Part model, mm, in its own coordinate system. Face numbers are marked on the shaded views. A direction names the side the tool comes from. Give positions to 0.01 mm unless a question says otherwise; leave off trailing zeros. Write each loop counter-clockwise with the first axis right and the second up, starting at its lowest first coordinate (ties: lowest second). Pieces come first, ordered by that corner, then holes. Notation, with made-up numbers: M -29,-19.75 L -17,-19.75 A22 cw -17,0.25 Z; hole C 66,-30 d9. An arc over 180 degrees is marked long. Answer as CSV lines item,"result". Start each with the question number.
Item 1: Band-saw the part on C-C, the plane z = -19.5. List the corners of the cut face in (x, y), then the cut area to 3 significant figures.
Item 2: Band-saw the part on D-D, the plane z = 14. List the corners of the cut face in (x, y), then the cut area to 3 significant figures.
Item 3: 3-axis set-ups, long thin cutter, end or side, ignore diameter. For the marked faces 4, 5 and 6: which of +Z, -Z, +X, -X, +Y, -Y reach the whole face in a straight line?
Item 4: Two-plate mould, pull along X, no slides. Class the marked faces 1, 2 and 3: +X half, -X half, draft (parallel to the pull), parting line (faces both ways), or undercut.
Item 5: Pin check, flat tips, straight feed: pin 1 (4 mm diameter, centred on x = 104.5, y = 0.5, fed in from +Z); pin 2 (1.2 mm diameter, centred on x = 89.5, y = -1.5, fed in from +Z); pin 3 (3 mm diameter, centred on y = -1.5, z = 1, fed in from +X); pin 4 (3 mm diameter, centred on x = 84, y = -0.5, fed in from +Z). Stop position of each tip, or through.
Item 6: Band-saw the part on B-B, the plane y = 2. List the corners of the cut face in (x, z) (3 decimals), then the cut area to 3 significant figures.
Item 7: Wall check: L1, parallel to X at y = 1.5, z = -7; L2, parallel to Z at x = 100, y = -1; L3, parallel to Y at x = 92, z = -19. Give the ranges that are in metal, low to high. Write a range as from..to.
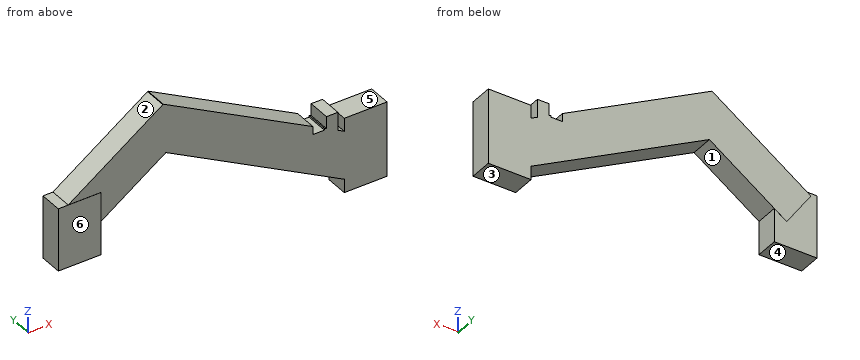
from build123d import *

# Parameters (mm, degrees)
F4_W      = 8
F4_H      = 15
F5_DEPTH  = 41.9
F6_W      = 8
F6_H      = 15
F7_DEPTH  = 84.2
F8_DEPTH  = 4.9
F9_W      = 15
F9_H      = 8
F10_DEPTH = 15.3
F11_DEPTH = 6.8
F12_W     = 15
F12_H     = 8
F13_DEPTH = 26.4
F14_W     = 4
F14_H     = 8
F15_DEPTH = 1.5
F16_W     = 4
F16_H     = 8
F17_DEPTH = 5
F18_DEPTH = 3


with BuildPart() as f5:
    # F4 (on face) → F5 (new body)
    with BuildSketch(Plane(origin=(-0.447452, 0, -0.306762), x_dir=(0, 1, 0), z_dir=(0.824783, 0, 0.56545))):
        Rectangle(F4_W, F4_H)
    extrude(amount=F5_DEPTH)

    # F6 (on face) → F7 (join)
    with BuildSketch(Plane(origin=(15.159437, 0, -8.175749), x_dir=(0, -1, 0), z_dir=(-0.880156, 0, 0.474684))):
        with Locations((0, 32.858156)):
            Rectangle(F6_W, F6_H)
    extrude(amount=-F7_DEPTH)

    # F6 (on face) → F8 (join)
    with BuildSketch(Plane(origin=(15.159437, 0, -8.175749), x_dir=(0, -1, 0), z_dir=(-0.880156, 0, 0.474684))):
        with Locations((0, 32.858156)):
            Rectangle(F6_W, F6_H)
    extrude(amount=F8_DEPTH)

    # F9 (on Top) → F10 (join)
    with BuildSketch(Plane.XY):
        with Locations((0.658734, -0.029655)):
            Rectangle(F9_W, F9_H)
    extrude(amount=-F10_DEPTH)

    # F9 (on Top) → F11 (join)
    with BuildSketch(Plane.XY):
        with Locations((0.658734, -0.029655)):
            Rectangle(F9_W, F9_H)
    extrude(amount=F11_DEPTH)

    # F12 (on Top) → F13 (join)
    with BuildSketch(Plane.XY):
        with Locations((101.044647, 0)):
            Rectangle(F12_W, F12_H)
    extrude(amount=-F13_DEPTH)

    # F14 (on Top) → F15 (cut, symmetric)
    with BuildSketch(Plane.XY):
        with Locations((84.574081, 0)):
            Rectangle(F14_W, F14_H)
    extrude(amount=F15_DEPTH, both=True, mode=Mode.SUBTRACT)

    # F16 (on Top) → F17 (join)
    with BuildSketch(Plane.XY):
        with Locations((89.305073, 0)):
            Rectangle(F16_W, F16_H)
    extrude(amount=-F17_DEPTH)

    # F16 (on Top) → F18 (join)
    with BuildSketch(Plane.XY):
        with Locations((89.305073, 0)):
            Rectangle(F16_W, F16_H)
    extrude(amount=F18_DEPTH)


solid = f5.part
Output:
1,outline,"M 89.58,-4 L 108.54,-4 L 108.54,4 L 89.58,4 Z"
1,area,"152 mm²"
2,outline,"M 7.16,-4 L 59.06,-4 L 59.06,4 L 7.16,4 Z"
2,area,"415 mm²"
3,face 4,"-Z, -X, +Y, -Y"
3,face 5,"+Z, +X, +Y, -Y"
3,face 6,"+Z, -Z, +X, -X, -Y"
4,face 1,"undercut"
4,face 2,"-X half"
4,face 3,"draft"
5,pin 1,"z = 0"
5,pin 2,"z = 3"
5,pin 3,"x = 108.54"
5,pin 4,"z = 1.36"
6,outline,"M -6.841,-15.3 L 8.159,-15.3 L 8.159,-3.5 L 30.945,12.122 L 93.545,-21.639 L 93.545,-26.4 L 108.545,-26.4 L 108.545,0 L 93.545,0 L 93.545,-4.597 L 91.305,-3.389 L 91.305,3 L 87.305,3 L 87.305,-1.232 L 86.574,-0.838 L 86.574,-1.5 L 82.574,-1.5 L 82.574,1.32 L 30.004,29.672 L 29.915,29.506 L 29.87,29.571 L -3.345,6.8 L -6.841,6.8 Z"
6,area,"2,270 mm²"
7,L1,"-6.84..8.16, 66.4..108.54"
7,L2,"-26.4..0"
7,L3,"-4..4"
